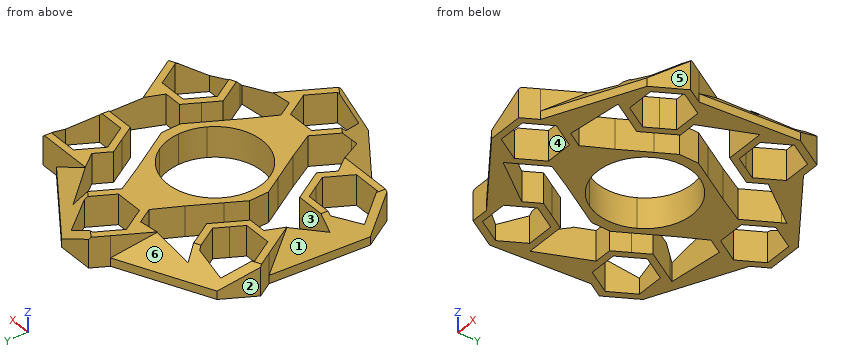
```python
from build123d import *

# Parameters (mm, degrees)
F1_DEPTH     = 6.9977
F2_T4_DEPTH  = 48.1283993469
F2_T9_DEPTH  = 48.1283993469
F2_T14_DEPTH = 48.1283993469
F2_T19_DEPTH = 48.1283993469
F2_T24_DEPTH = 48.1283993469
F2_T29_DEPTH = 48.1283993469
F3_SIZE      = 2.54


# Not quite as in the source:
# - a fillet or chamfer that OpenCascade refuses, or shapes differently, is made with other operations: its cross-section is extruded or revolved along the edge and cut away or added
# - a feature names something its author has since deleted; it is built from what else it names


with BuildPart() as f1:
    # F0 (on Top) → F1 (new body)
    with BuildSketch(Plane.XY):
        Polygon((-13.9314619955, -12.7), (-15.9478578107, -9.2075), (-17.9642536258, -5.715), (-26.0298368864, -5.715), (-30.0626285167, -12.7), (-26.0298368864, -19.685), (-21.9970452561, -19.685), (-17.9642536258, -19.685), (-15.9478578107, -16.1925), align=None)
        Polygon((-18.8441354361, -7.239), (-17.2676805261, -9.9695), (-15.691225616, -12.7), (-18.8441354361, -18.161), (-25.1499550762, -18.161), (-28.3028648962, -12.7), (-25.1499550762, -7.239), align=None, mode=Mode.SUBTRACT)
        with BuildLine():
            ThreePointArc((-9.4807265054, -5.4737), (-10.9474, 0), (-9.4807265054, 5.4737))
            Line((-9.4807265054, 5.4737), (-10.8318467228, 6.2537696213))
            Line((-10.8318467228, 6.2537696213), (-14.4424622971, 0))
            Line((-14.4424622971, 0), (-10.8318467228, -6.2537696213))
            Line((-10.8318467228, -6.2537696213), (-9.4807265054, -5.4737))
        make_face()
        Polygon((-17.9642536258, 5.715), (-15.9478578107, 9.2075), (-13.9314619955, 12.7), (-17.9642536258, 19.685), (-26.0298368864, 19.685), (-30.0626285167, 12.7), (-28.0462327016, 9.2075), (-26.0298368864, 5.715), (-21.9970452561, 5.715), align=None)
        Polygon((-15.691225616, 12.7), (-17.2676805261, 9.9695), (-18.8441354361, 7.239), (-25.1499550762, 7.239), (-28.3028648962, 12.7), (-25.1499550762, 18.161), (-18.8441354361, 18.161), align=None, mode=Mode.SUBTRACT)
        Polygon((-27.0032693489, -5.715), (-21.9970452561, 5.715), (-26.0298368864, 5.715), (-28.0462327016, 9.2075), (-30.0626285167, -12.7), align=None)
        Polygon((-18.4509698571, 20.5280172414), (-6.0491874454, 21.9075), (-8.0655832606, 25.4), (-6.0491874454, 28.8925), (-26.0298368864, 19.685), align=None)
        Polygon((-4.0327916303, 18.415), (4.0327916303, 18.415), (8.0655832606, 25.4), (4.0327916303, 32.385), (-4.0327916303, 32.385), (-6.0491874454, 28.8925), (-8.0655832606, 25.4), (-6.0491874454, 21.9075), align=None)
        Polygon((-6.3058196401, 25.4), (-3.15290982, 30.861), (3.15290982, 30.861), (6.3058196401, 25.4), (3.15290982, 19.939), (-3.15290982, 19.939), align=None, mode=Mode.SUBTRACT)
        Polygon((8.5522994918, 26.2430172414), (15.9478578107, 16.1925), (17.9642536258, 19.685), (21.9970452561, 19.685), (4.0327916303, 32.385), align=None)
        Polygon((27.0032693489, 5.715), (21.9970452561, -5.715), (26.0298368864, -5.715), (28.0462327016, -9.2075), (30.0626285167, 12.7), align=None)
        Polygon((13.9314619955, 12.7), (15.9478578107, 9.2075), (17.9642536258, 5.715), (26.0298368864, 5.715), (30.0626285167, 12.7), (26.0298368864, 19.685), (21.9970452561, 19.685), (17.9642536258, 19.685), (15.9478578107, 16.1925), align=None)
        Polygon((18.8441354361, 7.239), (17.2676805261, 9.9695), (15.691225616, 12.7), (18.8441354361, 18.161), (25.1499550762, 18.161), (28.3028648962, 12.7), (25.1499550762, 7.239), align=None, mode=Mode.SUBTRACT)
        Polygon((18.4509698571, -20.5280172414), (6.0491874454, -21.9075), (8.0655832606, -25.4), (6.0491874454, -28.8925), (26.0298368864, -19.685), align=None)
        Polygon((6.0491874454, -21.9075), (4.0327916303, -18.415), (-4.0327916303, -18.415), (-8.0655832606, -25.4), (-4.0327916303, -32.385), (4.0327916303, -32.385), (6.0491874454, -28.8925), (8.0655832606, -25.4), align=None)
        Polygon((-6.3058196401, -25.4), (-3.15290982, -19.939), (3.15290982, -19.939), (6.3058196401, -25.4), (3.15290982, -30.861), (-3.15290982, -30.861), align=None, mode=Mode.SUBTRACT)
        Polygon((-8.5522994918, -26.2430172414), (-15.9478578107, -16.1925), (-17.9642536258, -19.685), (-21.9970452561, -19.685), (-4.0327916303, -32.385), align=None)
        with BuildLine():
            Line((10.8318467228, -6.2537696213), (9.4807265054, -5.4737))
            ThreePointArc((9.4807265054, -5.4737), (0, -10.9474), (-9.4807265054, -5.4737))
            Line((-9.4807265054, -5.4737), (-10.8318467228, -6.2537696213))
            Line((-10.8318467228, -6.2537696213), (-7.2212311486, -12.5075392425))
            Line((-7.2212311486, -12.5075392425), (7.2212311486, -12.5075392425))
            Line((7.2212311486, -12.5075392425), (10.8318467228, -6.2537696213))
        make_face()
        with BuildLine():
            ThreePointArc((9.4807265054, 5.4737), (10.5743763907, 2.8333956144), (10.9474, 0))
            ThreePointArc((10.9474, 0), (10.5743763907, -2.8333956144), (9.4807265054, -5.4737))
            Line((9.4807265054, -5.4737), (10.8318467228, -6.2537696213))
            Line((10.8318467228, -6.2537696213), (14.4424622971, 0))
            Line((14.4424622971, 0), (10.8318467228, 6.2537696213))
            Line((10.8318467228, 6.2537696213), (9.4807265054, 5.4737))
        make_face()
        with BuildLine():
            ThreePointArc((-9.4807265054, 5.4737), (0, 10.9474), (9.4807265054, 5.4737))
            Line((9.4807265054, 5.4737), (10.8318467228, 6.2537696213))
            Line((10.8318467228, 6.2537696213), (7.2212311486, 12.5075392425))
            Line((7.2212311486, 12.5075392425), (-7.2212311486, 12.5075392425))
            Line((-7.2212311486, 12.5075392425), (-10.8318467228, 6.2537696213))
            Line((-10.8318467228, 6.2537696213), (-9.4807265054, 5.4737))
        make_face()
        Polygon((17.9642536258, -5.715), (15.9478578107, -9.2075), (13.9314619955, -12.7), (17.9642536258, -19.685), (26.0298368864, -19.685), (30.0626285167, -12.7), (28.0462327016, -9.2075), (26.0298368864, -5.715), (21.9970452561, -5.715), align=None)
        Polygon((15.691225616, -12.7), (17.2676805261, -9.9695), (18.8441354361, -7.239), (25.1499550762, -7.239), (28.3028648962, -12.7), (25.1499550762, -18.161), (18.8441354361, -18.161), align=None, mode=Mode.SUBTRACT)
        Polygon((-26.0298368864, 19.685), (-17.9642536258, 19.685), (-18.4509698571, 20.5280172414), align=None)
        Polygon((30.0626285167, 12.7), (26.0298368864, 5.715), (27.0032693489, 5.715), align=None)
        Polygon((26.0298368864, -19.685), (17.9642536258, -19.685), (18.4509698571, -20.5280172414), align=None)
        Polygon((-30.0626285167, -12.7), (-26.0298368864, -5.715), (-27.0032693489, -5.715), align=None)
        Polygon((-7.2212311486, 12.5075392425), (7.2212311486, 12.5075392425), (4.0327916303, 18.415), (-4.0327916303, 18.415), align=None)
        Polygon((4.0327916303, -18.415), (7.2212311486, -12.5075392425), (-7.2212311486, -12.5075392425), (-4.0327916303, -18.415), align=None)
        Polygon((-4.0327916303, -32.385), (-8.0655832606, -25.4), (-8.5522994918, -26.2430172414), align=None)
        Polygon((4.0327916303, 32.385), (8.0655832606, 25.4), (8.5522994918, 26.2430172414), align=None)
    extrude(amount=F1_DEPTH)

    # F2: chamfer of 5.08 on 6 edges, made by hand


with BuildPart() as f2_tool2:
    # F2_s3 → F2_t4 (new body)
    with BuildSketch(Plane(origin=(-1.8021315116, -19.5795864057, 0), x_dir=(0, 0, 1), z_dir=(0.0916539378, 0.9957909197, 0))):
        Polygon((1.9177, 28.7720874875), (6.9977, 23.6920874875), (6.9977, 28.7720874875), align=None)
    extrude(amount=F2_T4_DEPTH)

    split(bisect_by=Plane(origin=(17.0477100735, 9.8425, 0), x_dir=(0, 0, 1), z_dir=(0.8660254038, 0.5, 0)), keep=Keep.TOP)


with BuildPart() as f1_1:
    add(f1.part)

    # F2_t1: cut F2_tool2
    add(f2_tool2.part, mode=Mode.SUBTRACT)


with BuildPart() as f2_tool7:
    # F2_s8 → F2_t9 (new body)
    with BuildSketch(Plane(origin=(16.0553534671, -11.3504848729, 0), x_dir=(0, 0, 1), z_dir=(-0.8165532644, 0.5772700984, 0))):
        Polygon((1.9177, 28.7720874875), (6.9977, 23.6920874875), (6.9977, 28.7720874875), align=None)
    extrude(amount=F2_T9_DEPTH)

    split(bisect_by=Plane.XZ.offset(-19.685), keep=Keep.BOTTOM)


with BuildPart() as f1_2:
    add(f1_1.part)

    # F2_t6: cut F2_tool7
    add(f2_tool7.part, mode=Mode.SUBTRACT)


with BuildPart() as f2_tool12:
    # F2_s13 → F2_t14 (new body)
    with BuildSketch(Plane(origin=(17.8574849787, 8.2291015328, 0), x_dir=(0, 0, 1), z_dir=(-0.9082072022, -0.4185208213, 0))):
        Polygon((1.9177, 28.7720874875), (6.9977, 23.6920874875), (6.9977, 28.7720874875), align=None)
    extrude(amount=F2_T14_DEPTH)

    split(bisect_by=Plane(origin=(-17.0477100735, 9.8425, 0), x_dir=(0, 0, 1), z_dir=(-0.8660254038, 0.5, 0)), keep=Keep.TOP)


with BuildPart() as f1_3:
    add(f1_2.part)

    # F2_t11: cut F2_tool12
    add(f2_tool12.part, mode=Mode.SUBTRACT)


with BuildPart() as f2_tool17:
    # F2_s18 → F2_t19 (new body)
    with BuildSketch(Plane(origin=(1.8021315116, 19.5795864057, 0), x_dir=(0, 0, 1), z_dir=(-0.0916539378, -0.9957909197, 0))):
        Polygon((1.9177, 28.7720874875), (6.9977, 23.6920874875), (6.9977, 28.7720874875), align=None)
    extrude(amount=F2_T19_DEPTH)

    split(bisect_by=Plane(origin=(-17.0477100735, -9.8425, 0), x_dir=(0, 0, 1), z_dir=(-0.8660254038, -0.5, 0)), keep=Keep.TOP)


with BuildPart() as f1_4:
    add(f1_3.part)

    # F2_t16: cut F2_tool17
    add(f2_tool17.part, mode=Mode.SUBTRACT)


with BuildPart() as f2_tool22:
    # F2_s23 → F2_t24 (new body)
    with BuildSketch(Plane(origin=(-16.0553534671, 11.3504848729, 0), x_dir=(0, 0, 1), z_dir=(0.8165532644, -0.5772700984, 0))):
        Polygon((1.9177, 28.7720874875), (6.9977, 23.6920874875), (6.9977, 28.7720874875), align=None)
    extrude(amount=F2_T24_DEPTH)

    split(bisect_by=Plane.XZ.offset(19.685), keep=Keep.TOP)


with BuildPart() as f1_5:
    add(f1_4.part)

    # F2_t21: cut F2_tool22
    add(f2_tool22.part, mode=Mode.SUBTRACT)


with BuildPart() as f2_tool27:
    # F2_s28 → F2_t29 (new body)
    with BuildSketch(Plane(origin=(-17.8574849787, -8.2291015328, 0), x_dir=(0, 0, 1), z_dir=(0.9082072022, 0.4185208213, 0))):
        Polygon((1.9177, 28.7720874875), (6.9977, 23.6920874875), (6.9977, 28.7720874875), align=None)
    extrude(amount=F2_T29_DEPTH)

    split(bisect_by=Plane(origin=(17.0477100735, -9.8425, 0), x_dir=(0, 0, 1), z_dir=(0.8660254038, -0.5, 0)), keep=Keep.TOP)


with BuildPart() as f1_6:
    add(f1_5.part)

    # F2_t26: cut F2_tool27
    add(f2_tool27.part, mode=Mode.SUBTRACT)

    # F3
    f3_edges = [f1_6.edges().sort_by_distance(p)[0] for p in [
        (-14.442462, 0, 3.49885),
        (14.442462, 0, 3.49885),
    ]]
    chamfer(f3_edges, length=F3_SIZE)


solid = f1_6.part
```
Part model, mm, in its own coordinate system. Face numbers are marked on the shaded views. A direction names the side the tool comes from. Coordinates: 2 decimals unless noted, no trailing zeros. Order: outer loops, then holes, each group sorted by start corner. A loop starts at its lowest first (then second) coordinate and runs counter-clockwise, first axis right, second up. Notation, with made-up numbers: (53, 23) - (97, 23) arc R22 cw to (97, 35) - close; hole circle Ø1 at (55, 42.5). An arc over 180 degrees is marked (long way). Return JSON: item names as keys, results as strings. Group by question number.
Item 1: Drill centre lines: probe 1 along Y at (x, z) = (8, 1); probe 2 along Y at (x, z) = (-1, 2) (3 decimals); probe 3 along X at (y, z) = (-12, 2.5). Where is each one in solid material? Low to high. Write a range as from..to.
Item 2: Cut at D-D (z = 0.75). State how many separate pieces and enclosed holes the cut face has, plus the area to 3 significant figures.
Item 3: Pull direction Y, two halves, no side cores. Call the marked faces 4, 5 and 6: pulls with the +Y half, pulls with the -Y half, needs draft (parallel to the pull), parting line crosses it, or undercut.
Item 4: Which spindle directions (+Z, -Z, +X, -X, +Y, -Y) get a long thin tool onto all of the face, cutting with end or side? Do the marked faces 1, 2 and 3. Say none if no direction does.
Item 5: Cut at B-B (x = 12). List the corners of the cut face in (y, z), plus the area to 3 significant figures.
Item 6: Cut at C-C (y = 3). List the corners of the cut face in (x, z).
Item 7: Cut at A-A (x = 0.5). List the corners of the cut face in (y, z) (1 decimal), plus the area to 3 significant figures.
Item 8: Pin check, flat tips, straight feed: pin 1 (1.9 mm diameter, centred on x = 20.5, z = 3.5, fed in from +Y); pin 2 (1.9 mm diameter, centred on x = 21, z = 3, fed in from -Y); pin 3 (2 mm diameter, centred on x = -20.5, z = 3, fed in from -Y); pin 4 (4 mm diameter, centred on x = 3, y = -13.5, fed in from -Z). Stop position of each tip, or through.
Check values:
{
 "1": {"probe 1": "y = -27.99..-21.69, -11.16..-7.47, 7.47..11.16, 25.29..29.58", "probe 2": "y = -32.385..-30.861, -19.939..-10.902, 10.902..19.939, 30.861..32.385", "probe 3": "x = -29.41..-27.9, -16.1..-14.34, -7.51..7.51, 14.34..16.1, 27.9..29.66"},
 "2": {"separate pieces": "1", "enclosed holes": "9", "area": "1,080 mm2"},
 "3": {"face 4": "undercut", "face 5": "pulls with the -Y half", "face 6": "pulls with the +Y half"},
 "4": {"face 1": "+Z, -X", "face 2": "+Z, -Z, -X, +Y", "face 3": "+Z, -Z"},
 "5": {"outline": "(-26.15, 0) - (-21.25, 0) - (-21.25, 6.37) - (-26.15, 1.92) - close; (-4.23, 0) - (4.23, 0) - (4.23, 7) - (-4.23, 7) - close; (21.56, 0) - (26.75, 0) - (26.75, 1.92) - (21.56, 6.16) - close", "area": "101 mm2"},
 "6": {"outline": "(-28.62, 0) - (-23.19, 0) - (-23.19, 7) - (-24.46, 7) - (-24.46, 6.06) - (-28.62, 1.92) - close; (-12.71, 0) - (-10.53, 0) - (-10.53, 7) - (-12.71, 7) - close; (10.53, 0) - (12.71, 0) - (12.71, 7) - (10.53, 7) - close; (25.81, 0) - (29.17, 0) - (29.17, 1.92) - (25.81, 5.26) - close"},
 "7": {"outline": "(-32.4, 0) - (-30.9, 0) - (-30.9, 5.8) - (-32.4, 4.5) - close; (-19.9, 0) - (-10.9, 0) - (-10.9, 7) - (-19.9, 7) - close; (10.9, 0) - (19.9, 0) - (19.9, 7) - (10.9, 7) - close; (30.9, 0) - (32.4, 0) - (32.4, 4) - (30.9, 5.2) - close", "area": "141 mm2"},
 "8": {"pin 1": "stops at y = 20.15", "pin 2": "stops at y = -21.95", "pin 3": "stops at y = -20.83", "pin 4": "stops at z = 0"}
}
